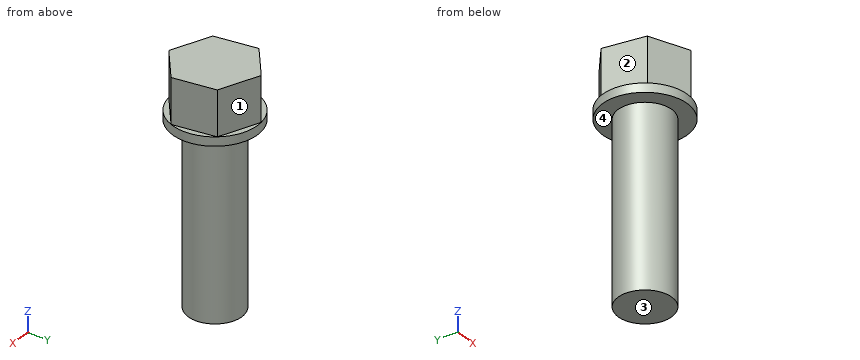
from build123d import *

# Parameters (mm, degrees)
CROQUIS1_R              = 6
SALIENTE_EXTRUIR1_DEPTH = 40
CROQUIS2_R              = 9.5
SALIENTE_EXTRUIR2_DEPTH = 2
SALIENTE_EXTRUIR3_DEPTH = 10


with BuildPart() as part:
    # Croquis1 → Saliente-Extruir1 (new body)
    with BuildSketch(Plane.XY):
        Circle(CROQUIS1_R)
    extrude(amount=SALIENTE_EXTRUIR1_DEPTH)

    # Croquis2 → Saliente-Extruir2 (add)
    with BuildSketch(Plane.XY.offset(40)):
        Circle(CROQUIS2_R)
    extrude(amount=SALIENTE_EXTRUIR2_DEPTH)

    # Croquis3 → Saliente-Extruir3 (add)
    with BuildSketch(Plane.XY.offset(42)):
        Polygon((-1.344767868, 9.404339391), (-8.816780752, 3.53756656), (-7.472012885, -5.866772831), (1.344767868, -9.404339391), (8.816780752, -3.53756656), (7.472012885, 5.866772831), align=None)
    extrude(amount=SALIENTE_EXTRUIR3_DEPTH)


solid = part.part
Could you check a few things on this model? Use its own coordinates, in mm. Face numbers are marked on the shaded views. A direction names the side the tool comes from. Give positions to 0.01 mm unless a question says otherwise; leave off trailing zeros. Loops run counter-clockwise (first coordinate to the right, second up) from the corner with the lowest first, then second, coordinate; pieces in that order, holes last. Notation, with made-up numbers: (87.5, 21) -> (99.5, 21) arc R17 ccw to (99.5, 38) -> close; hole circle Ø3 at (34.5, -27.75). An arc over 180 degrees is marked (long way). Return JSON: item names as keys, results as strings.
Item 1: I need wall thicknesses on L1, parallel to X at y = 1.25, z = 22.5; L2, parallel to Z at x = 1.75, y = -7.75; L3, parallel to Z at x = 5, y = -7.5. Which ranges of each line are inside material? Lowest first, please. Write a range as from..to.
Geometry results:
{"L1": "x = -5.87..5.87", "L2": "z = 40..52", "L3": "z = 40..42"}
Item 2: Which directions (+Z, -Z, +X, -X, +Y, -Y) give clear straight access to the entire face, cutting with the end or side of a thin tool? Please do the marked faces 1, 2, 3 and 4.
Geometry results:
{"face 1": "+Z, +X, +Y", "face 2": "+Z, -X, -Y", "face 3": "-Z, +X, -X, +Y, -Y", "face 4": "-Z"}
Item 3: I'm going to push flat-ended pins straight in: pin 1 (1.1 mm diameter, centred on x = -4, y = -8.5, fed in from +Z); pin 2 (3 mm diameter, centred on x = -6.5, z = 21, fed in from +Y); pin 3 (2 mm diameter, centred on x = 4, z = 42.5, fed in from +Y); pin 4 (4 mm diameter, centred on x = 4, y = 2, fed in from -Z). Where does each tip first touch, or does it pass through?
Geometry results:
{"pin 1": "stops at z = 42", "pin 2": "stops at y = 3.32", "pin 3": "stops at y = 8.97", "pin 4": "stops at z = 0"}
Item 4: If we section it at A-A on y = 0: List the corners of the cut face in (x, z) for me.
Geometry results:
{"outline": "(-9.5, 40) -> (-6, 40) -> (-6, 0) -> (6, 0) -> (6, 40) -> (9.5, 40) -> (9.5, 42) -> (8.31, 42) -> (8.31, 52) -> (-8.31, 52) -> (-8.31, 42) -> (-9.5, 42) -> close"}
Item 5: If we section it at C-C on z = 21.5: List the corners of the cut face in (x, y) for me, plus the area to 3 significant figures.
Geometry results:
{"outline": "circle Ø12 at (0, 0)", "area": "113 mm²"}
Item 6: If we section it at B-B on x = 0: List the corners of the cut face in (y, z) for me, plus the area to 3 significant figures.
Geometry results:
{"outline": "(-9.5, 40) -> (-6, 40) -> (-6, 0) -> (6, 0) -> (6, 40) -> (9.5, 40) -> (9.5, 42) -> (8.86, 42) -> (8.86, 52) -> (-8.86, 52) -> (-8.86, 42) -> (-9.5, 42) -> close", "area": "695 mm²"}
Item 7: If we section it at D-D on y = 7: List the corners of the cut face in (x, z) for me.
Geometry results:
{"outline": "(-6.42, 40) -> (6.42, 40) -> (6.42, 42) -> (4.65, 42) -> (4.65, 52) -> (-4.41, 52) -> (-4.41, 42) -> (-6.42, 42) -> close"}
